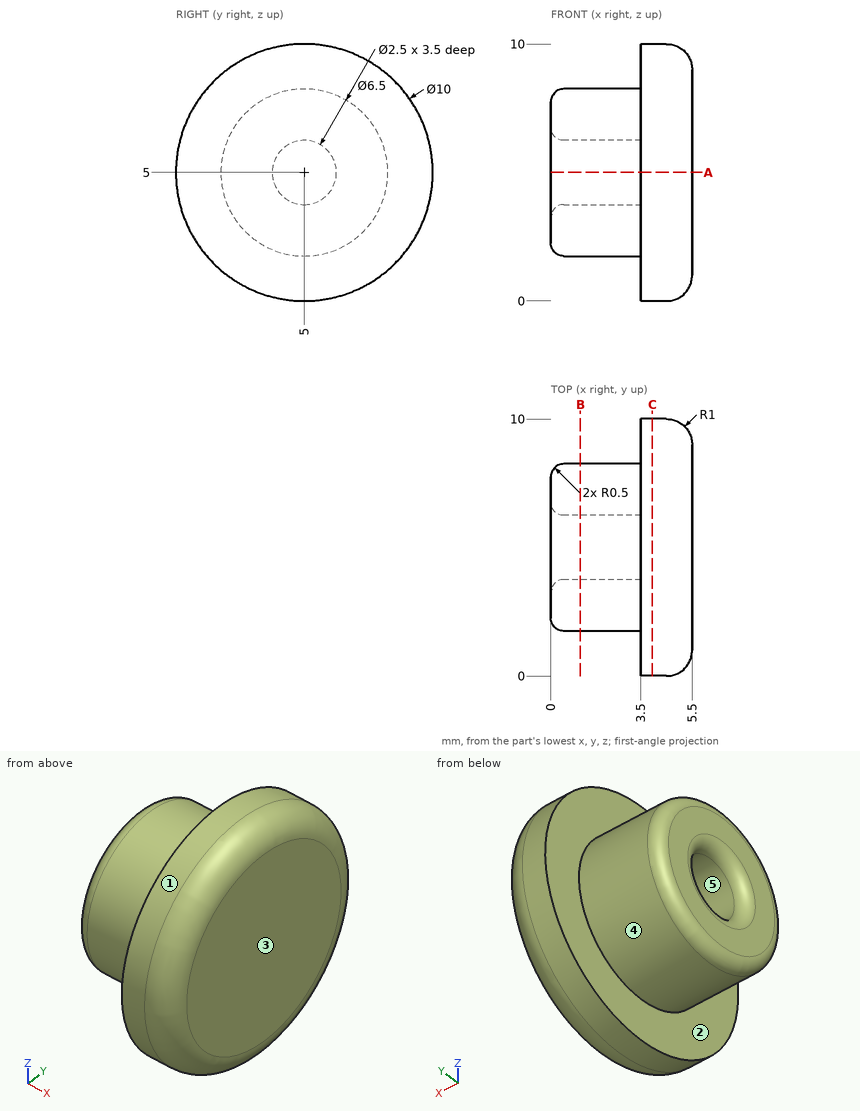
Could you check a few things on this drawing? It's one solid part, dimensions in mm from its lowest x, y, z. A direction names the side the tool comes from. Round coordinates to 2 decimals unless told otherwise and drop trailing zeros. Loops run counter-clockwise (first coordinate to the right, second up) from the corner with the lowest first, then second, coordinate; pieces in that order, holes last. Notation, with made-up numbers: M -2,35.25 L 13,35.25 A23 ccw 13,71.25 Z; hole C 77,42 d10. An arc over 180 degrees is marked long. Write each question's results on one line, items separated by ' | '. Start each with the question number.
(1) On a 3-axis mill with a long thin cutter (end or side, diameter ignored), from which of +Z, -Z, +X, -X, +Y, -Y can I reach the whole of each face in a straight line? I mean the marked faces 1 and 2. Say none if no direction works.
(2) Will these pins go through, and if not, where does the flat tip stop? P1, Ø3, axis at y = 5, z = 5, coming from the -X side; P2, Ø2, axis at x = 4, z = 2.5, coming from the +Y side; P3, Ø2, axis at x = 4.5, z = 3, coming from the +Y side.
(3) I want a section at C-C (x = 3.95). Please give me the cut outline in (y, z), then the cut area to 3 significant figures.
(4) I want a section at B-B (x = 1.15). Please give me the cut outline in (y, z).
(5) I want a section at A-A (z = 5). Please give me the cut outline in (x, y), then the cut area to 3 significant figures.
(6) Thinking about a two-plate mould opening in Z: for the marked faces 3, 4 and 5, which applies, pulls with the +Z half, pulls with the -Z half, needs draft (parallel to the pull), parting line crosses it, or undercut?
(7) If I drill on probe 1 along Y at (x, z) = (1.65, 5); probe 2 along Z at (x, y) = (1.9, 8); probe 3 along X at (y, z) = (5.5, 1), over which ranges is the centre line in solid material (lowest first)? Write a range as from..to.
Solved:
1) face 1: +X, -X | face 2: -X
2) P1: stops at x = 0.07 | P2: stops at y = 9.77 | P3: stops at y = 9.9
3) outline: C 5,5 d10 | area: 78.5 mm²
4) outline: C 5,5 d6.5; hole C 5,5 d2.5
5) outline: M 0,2.25 A0.5 ccw 0.5,1.75 L 3.5,1.75 L 3.5,0 L 4.5,0 A1 ccw 5.5,1 L 5.5,9 A1 ccw 4.5,10 L 3.5,10 L 3.5,8.25 L 0.5,8.25 A0.5 ccw 0,7.75 L 0,6.75 A0.5 ccw 0.5,6.25 L 3.5,6.25 L 3.5,3.75 L 0.5,3.75 A0.5 ccw 0,3.25 Z | area: 33.4 mm²
6) face 3: needs draft | face 4: parting line crosses it | face 5: undercut
7) probe 1: y = 1.75..3.75, 6.25..8.25 | probe 2: z = 3.75..6.25 | probe 3: x = 3.5..5.5
